```python
from build123d import *

# Parameters (mm, degrees)
CUT_EXTRUDE1_DEPTH      = 20.455471518
CUT_EXTRUDE1_DEPTH_BACK = 20.455471518
SKETCH2_W               = 1.1684
SKETCH2_H               = 0.7874


with BuildPart() as part:
    # Sketch1 → Revolve1 (revolve)
    with BuildSketch(Plane.XY, mode=Mode.PRIVATE) as revolve1_sk:
        with BuildLine():
            Line((0, 0), (0, 19.05))
            ThreePointArc((0, 19.05), (1.117279291, 18.67312328), (1.778, 17.696497855))
            Line((1.778, 17.696497855), (1.778, 9.652))
            Line((1.778, 9.652), (2.794, 9.652))
            Line((2.794, 9.652), (2.794, 0))
            Line((2.794, 0), (0, 0))
        make_face()
    revolve(revolve1_sk.sketch.rotate(Axis((0, 0, 0), (0, 1, 0)), 90), axis=Axis((0, 0, 0), (0, 1, 0)))

    # Sketch2 → Cut-Extrude1 (cut, two sides: drawn at the far end of the back side and taken through both)
    with BuildSketch(Plane.XY.offset(-CUT_EXTRUDE1_DEPTH_BACK)):
        with Locations((0, 0.3937)):
            Rectangle(SKETCH2_W, SKETCH2_H)
    extrude(amount=CUT_EXTRUDE1_DEPTH + CUT_EXTRUDE1_DEPTH_BACK, mode=Mode.SUBTRACT)


solid = part.part
```
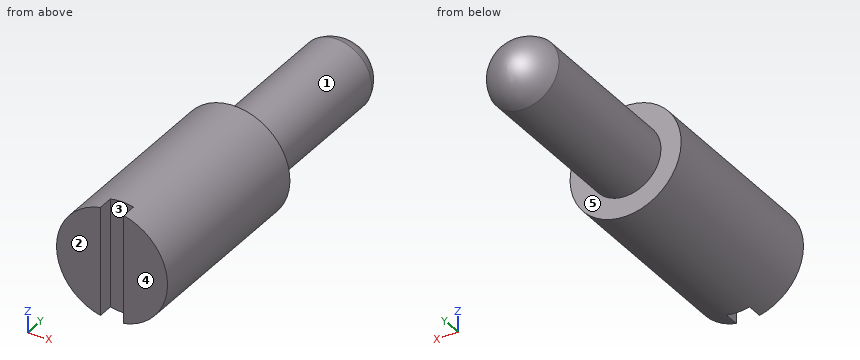
Here's how the part is built. I have some questions about the finished solid (model axes, mm). Face numbers are marked on the shaded views. A direction names the side the tool comes from. Give positions to 0.01 mm unless a question says otherwise; leave off trailing zeros. Write each loop counter-clockwise with the first axis right and the second up, starting at its lowest first coordinate (ties: lowest second). Pieces come first, ordered by that corner, then holes.
(1) Imagine slicing it at A-A, the plane z = 0. Write out the boundary of the cut face in (x, y), and give its area (3 significant figures).
Output values:
outline: (-2.79, 0) - (-0.58, 0) - (-0.58, 0.79) - (0.58, 0.79) - (0.58, 0) - (2.79, 0) - (2.79, 9.65) - (1.78, 9.65) - (1.78, 17.7) arc R1.84 ccw to (-1.78, 17.7) - (-1.78, 9.65) - (-2.79, 9.65) - close
area: 85.2 mm2
(2) Thinking about a two-plate mould opening in X: for the marked faces 1, 2 and 3, which applies, pulls with the +X half, pulls with the -X half, needs draft (parallel to the pull), parting line crosses it, or undercut?
Output values:
face 1: parting line crosses it
face 2: needs draft
face 3: undercut
(3) If I drill on L1, parallel to X at y = 2.5, z = 0.1; L2, parallel to Y at x = -1.8, z = 1.55, over which ranges is the centre line in solid material (lowest first)?
Output values:
L1: x = -2.79 to 2.79
L2: y = 0 to 9.65
(4) Will these pins go through, and if not, where does the flat tip stop? pin 1 (1.5 mm diameter, centred on x = -2, z = 0.5, fed in from +Y); pin 2 (3 mm diameter, centred on x = 2, z = -1.5, fed in from +Y); pin 3 (1.7 mm diameter, centred on x = -0.5, z = 1, fed in from +Y).
Output values:
pin 1: stops at y = 18.5
pin 2: stops at y = 18.76
pin 3: stops at y = 19.03
(5) Imagine slicing it at D-D, the plane x = -1.05. Write out the boundary of the cut face in (y, z), and give its area (3 significant figures).
Output values:
outline: (0, -2.59) - (9.65, -2.59) - (9.65, -1.43) - (17.7, -1.43) arc R1.52 ccw to (17.7, 1.43) - (9.65, 1.43) - (9.65, 2.59) - (0, 2.59) - close
area: 75.2 mm2
(6) Imagine slicing it at B-B, the plane x = 0. Write out the boundary of the cut face in (y, z), and give its area (3 significant figures).
Output values:
outline: (0.79, -2.79) - (9.65, -2.79) - (9.65, -1.78) - (17.7, -1.78) arc R1.84 ccw to (17.7, 1.78) - (9.65, 1.78) - (9.65, 2.79) - (0.79, 2.79) - close
area: 81.7 mm2
(7) On a 3-axis mill with a long thin cutter (end or side, diameter ignored), from which of +Z, -Z, +X, -X, +Y, -Y can I reach the whole of each face in a straight line? I mean the marked faces 4 and 5. Say none if no direction works.
Output values:
face 4: +Z, -Z, +X, -X, -Y
face 5: +Y
(8) Imagine slicing it at C-C, the plane y = 13.5. Write out the boundary of the cut face in (x, z), and give its area (3 significant figures).
Output values:
outline: circle Ø3.56 at (0, 0)
area: 9.93 mm2
